The listing builds one solid part. Answer for the finished solid, in the listing's coordinates (mm). A direction names the side the tool comes from. Give positions to 0.01 mm unless a question says otherwise; leave off trailing zeros. Order: outer loops, then holes, each group sorted by start corner. A loop starts at its lowest first (then second) coordinate and runs counter-clockwise, first axis right, second up. Notation, with made-up numbers: (-4.75, 56) - (24.25, 56) arc R27 cw to (24.25, 93) - close; hole circle Ø4 at (-6, 68). An arc over 180 degrees is marked (long way). Use a Markdown table: item, result. Add a question column.
1) For faces 5 (the face through (-1, 50.8, 13)), 6 (the face through (19.05, 0, 13)), determine the directions among +Z, -Z, +X, -X, +Y, -Y from which every point of the face is accessible in a straight line to the end or side of a thin tool.
2) The mould has two halves that part along X. Classify faces 1 (the face through (-50.8, -1, 13)), 2 (the face through (50.8, -1, 13)), 3 (the face through (22, 1, 0)), 4 (the face through (-19.05, 0, 13)): released by +X, released by -X, zero draft, split by the parting line, or undercut.
3) A flat-ended cylindrical pin translates along its axis: pin 1 (3 mm diameter, centred on x = -34, y = 36, fed in from -Z). Find the tip coordinate at first contact, or state that the pin passes through.
4) Find section D-D, the plane z = 6.5. Determine the outline of the cut face in (x, y).
5) Find section A-A, the plane y = 6.5. Determine the outline of the cut face in (x, z), plus the area to 3 significant figures.
6) Straight lines are drawn through the part: line 1 (X direction, y = 17.5, z = 2.25); line 2 (Y direction, x = -38.5, z = 23.75). For each, find the intervals that lie inside material, in ascending order.
7) Find section C-C, the plane y = -41. Determine the outline of the cut face in (x, z).
from build123d import *

# Parameters (mm, degrees)
F0_W     = 101.6
F0_H     = 101.6
F0_R     = 4.50054
F0_W_2   = 38.1
F0_H_2   = 38.1
F0_R_2   = 4.787872
F0_R_3   = 4.589665
F0_R_4   = 4.672002
F1_DEPTH = 25.4


with BuildPart() as f1:
    # F0 (on Top) → F1 (new body)
    with BuildSketch(Plane.XY):
        Rectangle(F0_W, F0_H)
        with Locations((-38.203955, -39.513808)):
            Circle(F0_R, mode=Mode.SUBTRACT)
        Rectangle(F0_W_2, F0_H_2, mode=Mode.SUBTRACT)
        with Locations((38.203955, -39.513808)):
            Circle(F0_R_2, mode=Mode.SUBTRACT)
        with Locations((-38.203955, 39.513808)):
            Circle(F0_R_3, mode=Mode.SUBTRACT)
        with Locations((38.203955, 39.513808)):
            Circle(F0_R_4, mode=Mode.SUBTRACT)
    extrude(amount=F1_DEPTH)


solid = f1.part
The answers:
| question | item | result |
|---|---|---|
| 1 | face 5 | +Z, -Z, +X, -X, +Y |
| 1 | face 6 | +Z, -Z |
| 2 | face 1 | released by -X |
| 2 | face 2 | released by +X |
| 2 | face 3 | zero draft |
| 2 | face 4 | undercut |
| 3 | pin 1 | z = 0 |
| 4 | outline | (-50.8, -50.8) - (50.8, -50.8) - (50.8, 50.8) - (-50.8, 50.8) - close; hole circle Ø9.18 at (-38.2, 39.51); hole circle Ø9 at (-38.2, -39.51); hole (-19.05, -19.05) - (19.05, -19.05) - (19.05, 19.05) - (-19.05, 19.05) - close; hole circle Ø9.58 at (38.2, -39.51); hole circle Ø9.34 at (38.2, 39.51) |
| 5 | outline | (-50.8, 0) - (-19.05, 0) - (-19.05, 25.4) - (-50.8, 25.4) - close; (19.05, 0) - (50.8, 0) - (50.8, 25.4) - (19.05, 25.4) - close |
| 5 | area | 1,610 mm2 |
| 6 | line 1 | -50.8 to -19.05, 19.05 to 50.8 |
| 6 | line 2 | -50.8 to -44, -35.02 to 34.93, 44.09 to 50.8 |
| 7 | outline | (-50.8, 0) - (-42.45, 0) - (-42.45, 25.4) - (-50.8, 25.4) - close; (-33.96, 0) - (33.65, 0) - (33.65, 25.4) - (-33.96, 25.4) - close; (42.76, 0) - (50.8, 0) - (50.8, 25.4) - (42.76, 25.4) - close |
